```python
from build123d import *

# Parameters (mm, degrees)
SKETCH_1_W          = 50
SKETCH_1_H          = 30
EXTRUDE_1_DEPTH     = 4
SKETCH_3_R          = 2.15
CUT_EXTRUDE_2_DEPTH = 4
SKETCH_4_R          = 1.6
CUT_EXTRUDE_3_DEPTH = 5
SKETCH_5_W          = 28
SKETCH_5_H          = 10
EXTRUDE_2_DEPTH     = 4
FILLET_1_R          = 1.5
FILLET_2_R          = 2


with BuildPart() as part:
    # 草图1 → 凸台-拉伸1 (new body)
    with BuildSketch(Plane.XY):
        with Locations((25, 15)):
            Rectangle(SKETCH_1_W, SKETCH_1_H)
    extrude(amount=EXTRUDE_1_DEPTH)

    # 草图3 → 切除-拉伸2 (cut)
    with BuildSketch(Plane.XY.offset(4)):
        with Locations((14.2, 18.9)):
            Circle(SKETCH_3_R)
        with Locations((35.8, 18.9)):
            Circle(SKETCH_3_R)
    extrude(amount=-CUT_EXTRUDE_2_DEPTH, mode=Mode.SUBTRACT)

    # 草图4 → 切除-拉伸3 (cut, through all)
    with BuildSketch(Plane.XY.offset(4)):
        with Locations((44, 7)):
            Circle(SKETCH_4_R)
        with Locations((6, 7)):
            Circle(SKETCH_4_R)
    extrude(amount=-CUT_EXTRUDE_3_DEPTH, mode=Mode.SUBTRACT)

    # 草图5 → 凸台-拉伸2 (add)
    with BuildSketch(Plane.XY.offset(4)):
        with Locations((25, -5)):
            Rectangle(SKETCH_5_W, SKETCH_5_H)
    extrude(amount=-EXTRUDE_2_DEPTH)

    # 圆角1
    fillet_1_edges = [part.edges().sort_by_distance(p)[0] for p in [
        (11, -10, 2),
        (39, -10, 2),
    ]]
    fillet(fillet_1_edges, radius=FILLET_1_R)

    # 圆角2
    fillet_2_edges = [part.edges().sort_by_distance(p)[0] for p in [
        (11, 0, 2),
        (39, 0, 2),
        (0, 30, 2),
        (50, 30, 2),
        (50, 0, 2),
        (0, 0, 2),
    ]]
    fillet(fillet_2_edges, radius=FILLET_2_R)


solid = part.part
```
CAD build for the part. Positions are in the model's coordinates, mm. A direction names the side the tool comes from. Round coordinates to 2 decimals unless told otherwise and drop trailing zeros. Order: outer loops, then holes, each group sorted by start corner. A loop starts at its lowest first (then second) coordinate and runs counter-clockwise, first axis right, second up. Notation, with made-up numbers: (81, 47.5) -> (94, 47.5) arc R9 cw to (94, 53.5) -> close; hole circle Ø11 at (68.5, -31). An arc over 180 degrees is marked (long way). One line per question, with ' | ' between items.
Q1. Two-plate mould, pull along Y, no slides. Class faces 1 (the flat face through (25, 10, 0)), 2 (the cylindrical face through (6.74, 5.58, 2.03)), 3 (the cylindrical face through (37.85, 19.55, 2.03)), 4 (the cylindrical face through (49.43, 0.6, 2.03)): released by +Y, released by -Y, zero draft, split by the parting line, or undercut.
Completed:
face 1: zero draft | face 2: undercut | face 3: undercut | face 4: released by -Y
Q2. Slice it at C-C (z = 1.2). Write the cut outline in (x, y).
Completed:
outline: (0, 2) arc R2 ccw to (2, 0) -> (9, 0) arc R2 cw to (11, -2) -> (11, -8.5) arc R1.5 ccw to (12.5, -10) -> (37.5, -10) arc R1.5 ccw to (39, -8.5) -> (39, -2) arc R2 cw to (41, 0) -> (48, 0) arc R2 ccw to (50, 2) -> (50, 28) arc R2 ccw to (48, 30) -> (2, 30) arc R2 ccw to (0, 28) -> close; hole circle Ø3.2 at (6, 7); hole circle Ø4.3 at (14.2, 18.9); hole circle Ø4.3 at (35.8, 18.9); hole circle Ø3.2 at (44, 7)
Q3. Slice it at B-B (x = 14.2). Write the cut outline in (y, z).
Completed:
outline: (-10, 0) -> (16.75, 0) -> (16.75, 4) -> (-10, 4) -> close; (21.05, 0) -> (30, 0) -> (30, 4) -> (21.05, 4) -> close
Q4. Slice it at D-D (x = 6). Write the cut outline in (y, z), then the cut area to 3 significant figures.
Completed:
outline: (0, 0) -> (5.4, 0) -> (5.4, 4) -> (0, 4) -> close; (8.6, 0) -> (30, 0) -> (30, 4) -> (8.6, 4) -> close | area: 107 mm^2
Q5. Drop flat-ended pins along their axis: pin 1 (2 mm diameter, centred on y = -4.5, z = 1, fed in from +X); pin 2 (2 mm diameter, centred on x = 46, z = 2, fed in from -Y). Give the stop position or say it passes through.
Completed:
pin 1: stops at x = 39 | pin 2: stops at y = 0
Q6. Probe probe 1 along Y at (x, z) = (44, 1.8); probe 2 along Y at (x, z) = (14.2, 2.3); probe 3 along Y at (x, z) = (8, 2.6). List the from-to ranges inside material, lowest first.
Completed:
probe 1: y = 0 to 5.4, 8.6 to 30 | probe 2: y = -10 to 16.75, 21.05 to 30 | probe 3: y = 0 to 30
Q7. Which spindle directions (+Z, -Z, +X, -X, +Y, -Y) get a long thin tool onto all of the face, cutting with end or side? Do faces 5 (the flat face through (5, 0, 2)), 6 (the flat face through (44, 0, 2)), 7 (the cylindrical face through (0.57, 29.4, 2.03)). Say none if no direction does.
Completed:
face 5: +Z, -Z, -X, -Y | face 6: +Z, -Z, +X, -Y | face 7: +Z, -Z, -X, +Y
Q8. Slice it at A-A (y = 18.9). Write the cut outline in (x, z).
Completed:
outline: (0, 0) -> (12.05, 0) -> (12.05, 4) -> (0, 4) -> close; (16.35, 0) -> (33.65, 0) -> (33.65, 4) -> (16.35, 4) -> close; (37.95, 0) -> (50, 0) -> (50, 4) -> (37.95, 4) -> close
